Source: CAD feature listing. Evaluate the final solid. Frame: model axes, mm. Give positions to 0.01 mm unless a question says otherwise; leave off trailing zeros. Order: outer loops, then holes, each group sorted by start corner. A loop starts at its lowest first (then second) coordinate and runs counter-clockwise, first axis right, second up. Notation, with made-up numbers: (-39.5, 45) -> (8.5, 45) arc R28 ccw to (8.5, 75) -> close; hole circle Ø3 at (88, 75). An arc over 180 degrees is marked (long way). Use one line per item in the form item = value. Start each with the question number.
Autodesk Inventor part; units mm, degrees
ref_plane "YZ Plane" through (0, 0, 0) normal (1, 0, 0) x (0, 1, 0)
ref_plane "XZ Plane" through (0, 0, 0) normal (0, 1, 0) x (-1, 0, 0)
ref_plane "XY Plane" through (0, 0, 0) normal (0, 0, 1) x (1, 0, 0)
sketch "Sketch1" plane through (0, 0, 0) normal (0, 0, 1) x (1, 0, 0)
  circle A0 centre (0, 0) radius 5.715
  circle A1 centre (203.2, 0) radius 2.1844
  line L0 (203.6465, -6.3343) -> (1.4511, -20.5864)
  circle A2 centre (1.7066, 23.2882) radius 2.1844
  circle A3 centre (-20.0159, 10.124) radius 2.1844
  line L1 (-23.3069, 15.5547) -> (-1.5845, 28.7188)
  line L2 (-25.8346, 7.5814) -> (-18.9109, -8.2635)
  arc A4 (-23.3069, 15.5547) -> (-25.8346, 7.5814) centre (-20.0159, 10.124) ccw
  line L3 (203.2, 6.35) -> (2.4369, 29.596)
  arc A5 (2.4369, 29.596) -> (-1.5845, 28.7188) centre (1.7066, 23.2882) ccw
  arc A6 (-18.9109, -8.2635) -> (1.4511, -20.5864) centre (0, 0) ccw
  circle A7 centre (14.3223, 21.8274) radius 2.1844
  circle A8 centre (77.2831, 14.5373) radius 2.1844
  circle A9 centre (140.2439, 7.2472) radius 2.1844
  circle A10 centre (35.0777, -11.8662) radius 2.1844
  circle A11 centre (102.3309, -7.1257) radius 2.1844
  arc A12 (203.6465, -6.3343) -> (203.2, 6.35) centre (203.2, 0) ccw
  dimension "d0" = 11.43
  dimension "d3" = 4.3688
  dimension "d30" = 4.3688
  dimension "d36" = 4.3688
  dimension "d45" = 4.3688
  dimension "d47" = 4.3688
  dimension "d51" = 4.3688
  dimension "d52" = 4.3688
extrude "Extrusion1" add sketch "Sketch1" along normal blind 1.5875
properties part number "intake"
1) Cut plane B-B, the plane z = 1.05. Count the separate pieces of the cut face and the enclosed holes in it, plus the area to 3 significant figures.
2) Draft query along X for faces 1 (the face through (104.22, 17.81, 0.78)), 2 (the face through (-22.42, -0.23, 0.78)), 3 (the face through (1.422, 21.122, 0.783)), 4 (the face through (64, 5, 0)). Return one class per face: +X half, -X half, draft (parallel to the pull), parting line (faces both ways), or undercut.
3) Cut plane D-D, the plane x = 164.5. Return the cut outline in (y, z).
4) Pin query (flat end, axial travel): pin 1 (2.5 mm diameter, centred on x = 1.71, y = 23.29, fed in from +Z). Return the tip coordinate at first contact, or that it passes through.
5) Cut plane A-A, the plane y = 0. Return the cut outline in (x, z) (1 decimal), plus the area to 3 significant figures.
6) Material intervals for probe 1 along Y at (x, z) = (203.2, 0.9); probe 2 along X at (y, z) = (-3.5, 1.35); probe 3 along X at (y, z) = (-4, 0.1), sorted ascending.
7) Cut plane C-C, the plane x = 112. Return the cut outline in (y, z).
Output values:
q1.separate_pieces = 1
q1.enclosed_holes = 9
q1.area = 7,160 mm^2
q2.face_1 = +X half
q2.face_2 = -X half
q2.face_3 = undercut
q2.face_4 = draft
q3.outline = (-9.09, 0) -> (10.83, 0) -> (10.83, 1.59) -> (-9.09, 1.59) -> close
q4.pin_1 = through
q5.outline = (-22.5, 0) -> (-5.7, 0) -> (-5.7, 1.6) -> (-22.5, 1.6) -> close; (5.7, 0) -> (201, 0) -> (201, 1.6) -> (5.7, 1.6) -> close; (205.4, 0) -> (209.6, 0) -> (209.6, 1.6) -> (205.4, 1.6) -> close
q5.area = 343 mm^2
q6.probe_1 = -6.37 to -2.18, 2.18 to 6.35
q6.probe_2 = -20.99 to -4.52, 4.52 to 208.5
q6.probe_3 = -20.77 to -4.08, 4.08 to 208.13
q7.outline = (-12.79, 0) -> (16.91, 0) -> (16.91, 1.59) -> (-12.79, 1.59) -> close
